Source: CAD feature listing. Evaluate the final solid. Frame: model axes, mm. Give positions to 0.01 mm unless a question says otherwise; leave off trailing zeros. Order: outer loops, then holes, each group sorted by start corner. A loop starts at its lowest first (then second) coordinate and runs counter-clockwise, first axis right, second up.
from build123d import *

# Parameters (mm, degrees)
F1_DEPTH = 6.35


with BuildPart() as f1:
    # F0 (on Top) → F1 (new body)
    with BuildSketch(Plane.XY):
        Polygon((-63.5, -88.9), (0, -88.9), (63.5, -88.9), (177.8, 88.9), (0, 88.9), (-177.8, 88.9), align=None)
        with BuildLine():
            ThreePointArc((0, -38.1), (-26.940768, 26.940768), (38.1, 0))
            ThreePointArc((38.1, 0), (26.940768, -26.940768), (0, -38.1))
        make_face(mode=Mode.SUBTRACT)
    extrude(amount=F1_DEPTH)


with BuildPart() as f2_1:
    # F2: copy of F1
    add(f1.part)


solid = f1.part
1) Section query B-B on y = 24. Output: boundary loops of the cut face in (x, z), and give its area (3 significant figures).
Checks:
outline: (-136.08, 0) - (-29.59, 0) - (-29.59, 6.35) - (-136.08, 6.35) - close; (29.59, 0) - (136.08, 0) - (136.08, 6.35) - (29.59, 6.35) - close
area: 1,350 mm2
2) Section query D-D on y = 70. Output: boundary loops of the cut face in (x, z), and give its area (3 significant figures).
Checks:
outline: (-165.65, 0) - (165.65, 0) - (165.65, 6.35) - (-165.65, 6.35) - close
area: 2,100 mm2
3) First-contact query: pin 1 Ø1.5 at (y, z) = (6, 5) entering from +X. Flat tip, straight axial feed; report the tip coordinate or a pass-through.
Checks:
pin 1: stops at x = 124.99
4) Ray query, L1, parallel to Y at x = -20, z = 0.75; L2, parallel to Y at x = 27, z = 3.5; L3, parallel to X at y = 65.5, z = 3.75. Return the intervals inside material, ascending.
Checks:
L1: y = -88.9 to -32.43, 32.43 to 88.9
L2: y = -88.9 to -26.88, 26.88 to 88.9
L3: x = -162.76 to 162.76
5) Section query C-C on x = 144.5. Output: boundary loops of the cut face in (y, z), and give its area (3 significant figures).
Checks:
outline: (37.1, 0) - (88.9, 0) - (88.9, 6.35) - (37.1, 6.35) - close
area: 329 mm2
6) Section query A-A on z = 4.25. Output: boundary loops of the cut face in (x, y).
Checks:
outline: (-177.8, 88.9) - (-63.5, -88.9) - (63.5, -88.9) - (177.8, 88.9) - close; hole (0, -38.1) arc R38.1 ccw to (38.1, 0) arc R38.1 ccw (long way) to start
